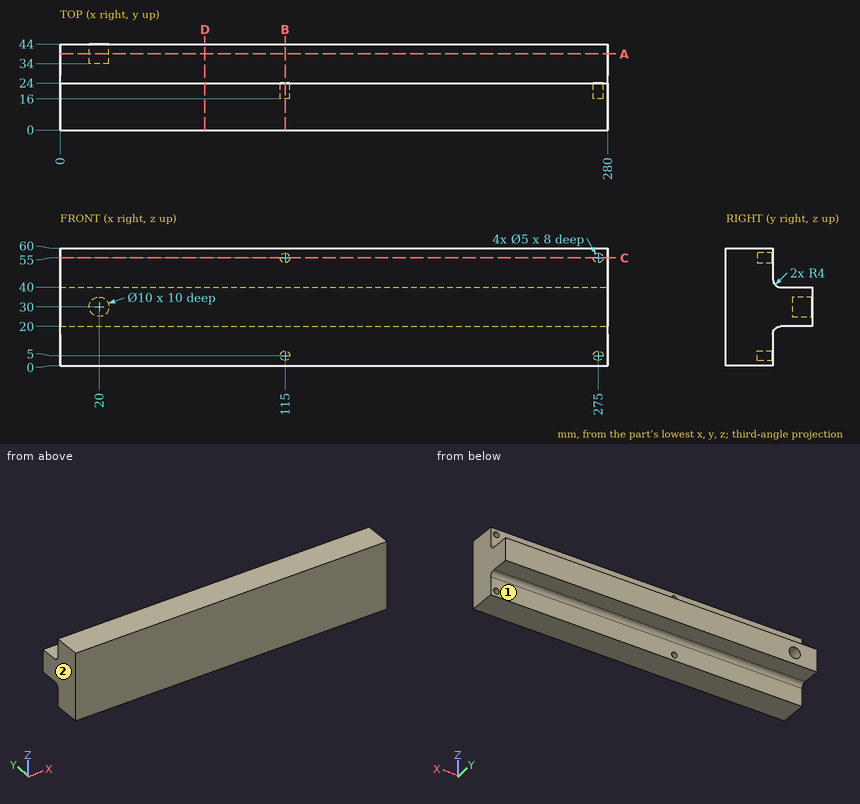
The drawing under review shows one solid part. Ordinate dimensions are in mm from its lowest x, y, z. A direction names the side the tool comes from. Give positions to 0.01 mm unless a question says otherwise; leave off trailing zeros. Order: outer loops, then holes, each group sorted by start corner. A loop starts at its lowest first (then second) coordinate and runs counter-clockwise, first axis right, second up. Notation, with made-up numbers: (2.25, 63.25) -> (59.25, 63.25) arc R17 cw to (59.25, 86.25) -> close; hole circle Ø3 at (77, -35.75). An arc over 180 degrees is marked (long way). Write item = value, one per line. Start each with the question number.
(1) To check wall thickness, follow line 1 along X through (y, z) = (17.75, 5); line 2 along Z through (x, y) = (275, 18); line 3 along Y through (x, z) = (24, 29). State the ranges of each line that lie inside material, in increasing order.
(2) For pin 1 (8 mm diameter, centred on x = 127, y = 32.5, fed in from -Z); pin 2 (13 mm diameter, centred on x = 200.5, z = 5, fed in from +Y); pin 3 (2.5 mm diameter, centred on x = 115.5, z = 4.5, fed in from +Y), all flat-tipped, find the tip position at first contact; note any pin that passes through.
(3) For the marked faces 1 and 2, list the 3-axis set-ups (+Z, -Z, +X, -X, +Y, -Y) from which the entire face can be reached by the end or side of a thin tool; tool diameter is ignored.
(4) We need section D-D on x = 74. Write out the cut boundary in (y, z).
(5) We need section C-C on z = 55. Write out the cut boundary in (x, y).
(6) We need section B-B on x = 115. Write out the cut boundary in (y, z).
(7) We need section A-A on y = 39. Write out the cut boundary in (x, z).
Numbers:
q1.line_1 = 0 to 112.5, 117.5 to 272.5, 277.5 to 280
q1.line_2 = 0 to 2.5, 7.5 to 52.5, 57.5 to 60
q1.line_3 = 0 to 34
q2.pin_1 = 20
q2.pin_2 = 24
q2.pin_3 = 16
q3.face_1 = -Z, +X, -X, +Y
q3.face_2 = +Z, -Z, -X, +Y, -Y
q4.outline = (0, 0) -> (24, 0) -> (24, 16) arc R4 cw to (28, 20) -> (44, 20) -> (44, 40) -> (28, 40) arc R4 cw to (24, 44) -> (24, 60) -> (0, 60) -> close
q5.outline = (0, 0) -> (280, 0) -> (280, 24) -> (277.5, 24) -> (277.5, 16) -> (272.5, 16) -> (272.5, 24) -> (117.5, 24) -> (117.5, 16) -> (112.5, 16) -> (112.5, 24) -> (0, 24) -> close
q6.outline = (0, 0) -> (24, 0) -> (24, 2.5) -> (16, 2.5) -> (16, 7.5) -> (24, 7.5) -> (24, 16) arc R4 cw to (28, 20) -> (44, 20) -> (44, 40) -> (28, 40) arc R4 cw to (24, 44) -> (24, 52.5) -> (16, 52.5) -> (16, 57.5) -> (24, 57.5) -> (24, 60) -> (0, 60) -> close
q7.outline = (0, 20) -> (280, 20) -> (280, 40) -> (0, 40) -> close; hole circle Ø10 at (20, 30)
